Input: part model. Units: mm. Frame: model coordinates. A direction names the side the tool comes from. Coordinates: 2 decimals unless noted, no trailing zeros. Loops run counter-clockwise (first coordinate to the right, second up) from the corner with the lowest first, then second, coordinate; pieces in that order, holes last.
Autodesk Inventor part; units mm, degrees
ref_plane "YZ Plane" through (0, 0, 0) normal (1, 0, 0) x (0, 1, 0)
ref_plane "XZ Plane" through (0, 0, 0) normal (0, 1, 0) x (-1, 0, 0)
ref_plane "XY Plane" through (0, 0, 0) normal (0, 0, 1) x (1, 0, 0)
sketch "Sketch1" plane through (0, 0, 0) normal (0, 1, 0) x (-1, 0, 0)
  line L0 (400, -50) -> (400, 50)
  line L1 (400, 50) -> (390, 50)
  line L2 (390, 50) -> (390, -40)
  line L3 (390, -40) -> (300, -40)
  line L4 (300, -40) -> (300, -50)
  line L5 (300, -50) -> (400, -50)
  line L6 (250, -50) -> (250, -40)
  line L7 (250, -40) -> (150, -40)
  line L8 (150, -40) -> (150, -50)
  line L9 (150, -50) -> (250, -50)
  line L10 (100, -50) -> (100, -40)
  line L11 (100, -40) -> (10, -40)
  line L12 (10, -40) -> (10, 50)
  line L13 (10, 50) -> (0, 50)
  line L14 (0, 50) -> (0, -50)
  line L15 (0, -50) -> (100, -50)
  point P0 (0, 0)
  dimension "d0" = 100
  dimension "d1" = 100
  dimension "d2" = 10
  dimension "d3" = 10
  dimension "d4" = 100
  dimension "d5" = 100
  dimension "d6" = 100
  dimension "d7" = 10
  dimension "d8" = 10
  dimension "d9" = 50
  dimension "d10" = 50
  dimension "d11" = 400
  dimension "d12" = 50
  dimension "d13" = 50
extrude "Extrusion1" add sketch "Sketch1" along normal blind 100
sketch "Sketch2" plane through (0, 0, 0) normal (1, 0, 0) x (0, 1, 0)
  point P0 (0, 0)
sketch "Sketch3" plane through (0, 0, 50) normal (1, 0, 0) x (0, 0, -1)
  line L0 (92.5, 80) -> (97.5, 80)
  line L1 (97.5, 80) -> (97.5, 75)
  line L2 (97.5, 75) -> (92.5, 75)
  line L3 (92.5, 75) -> (92.5, 80)
  line L4 (97.5, 20) -> (92.5, 20)
  line L5 (92.5, 20) -> (92.5, 25)
  line L6 (92.5, 25) -> (97.5, 25)
  line L7 (97.5, 25) -> (97.5, 20)
  line L8 (0, 100) -> (100, 100)
  line L9 (100, 0) -> (100, 100)
  line L10 (0, 0) -> (100, 0)
  line L11 (92.5, 52.5) -> (97.5, 52.5)
  line L12 (97.5, 52.5) -> (97.5, 47.5)
  line L13 (97.5, 47.5) -> (92.5, 47.5)
  line L14 (92.5, 47.5) -> (92.5, 52.5)
  point P0 (50, 0)
  dimension "d16" = 20
  dimension "d17" = 5
  dimension "d18" = 5
  dimension "d19" = 2.5
  dimension "d20" = 20
  dimension "d21" = 5
  dimension "d22" = 5
  dimension "d24" = 7.5
  dimension "d25" = 5
  dimension "d26" = 5
  dimension "d27" = 2.5
  dimension "d28" = 22.5
extrude "Extrusion2" cut sketch "Sketch3" against normal blind 320
sketch "Sketch4" plane through (0, 0, 50) normal (1, 0, 0) x (0, 0, -1)
  line L0 (97.5, 75) -> (92.5, 75)
  line L1 (97.5, 80) -> (97.5, 75)
  line L2 (92.5, 80) -> (97.5, 80)
  line L3 (92.5, 75) -> (92.5, 80)
  line L4 (97.5, 47.5) -> (92.5, 47.5)
  line L5 (97.5, 52.5) -> (97.5, 47.5)
  line L6 (92.5, 52.5) -> (97.5, 52.5)
  line L7 (92.5, 47.5) -> (92.5, 52.5)
  line L8 (92.5, 25) -> (97.5, 25)
  line L9 (92.5, 20) -> (92.5, 25)
  line L10 (97.5, 20) -> (92.5, 20)
  line L11 (97.5, 25) -> (97.5, 20)
  line L12 (92.5, 80) -> (97.5, 80)
  line L13 (97.5, 80) -> (97.5, 75)
  line L14 (97.5, 75) -> (92.5, 75)
  line L15 (92.5, 75) -> (92.5, 80)
  line L16 (92.5, 52.5) -> (97.5, 52.5)
  line L17 (97.5, 52.5) -> (97.5, 47.5)
  line L18 (97.5, 47.5) -> (92.5, 47.5)
  line L19 (92.5, 47.5) -> (92.5, 52.5)
  line L20 (92.5, 25) -> (97.5, 25)
  line L21 (97.5, 25) -> (97.5, 20)
  line L22 (97.5, 20) -> (92.5, 20)
  line L23 (92.5, 20) -> (92.5, 25)
  point P0 (50, 0)
extrude "Extrusion3" add sketch "Sketch4" against normal blind 80
sketch "Sketch6" plane through (-250, 0, -40) normal (0, 0, 1) x (1, 0, 0)
  line L0 (-50, 80) -> (-50, 75)
  line L1 (-50, 80) -> (-70, 80)
  line L2 (-70, 80) -> (-70, 75)
  line L3 (-50, 75) -> (-70, 75)
  line L4 (-50, 52.5) -> (-50, 47.5)
  line L5 (-50, 52.5) -> (-70, 52.5)
  line L6 (-70, 52.5) -> (-70, 47.5)
  line L7 (-50, 47.5) -> (-70, 47.5)
  line L8 (-50, 25) -> (-50, 20)
  line L9 (-50, 25) -> (-70, 25)
  line L10 (-70, 25) -> (-70, 20)
  line L11 (-50, 20) -> (-70, 20)
  line L12 (0, 75) -> (0, 80)
  line L13 (100, 75) -> (0, 75)
  line L14 (100, 80) -> (100, 75)
  line L15 (100, 80) -> (0, 80)
  line L16 (0, 47.5) -> (0, 52.5)
  line L17 (100, 47.5) -> (0, 47.5)
  line L18 (100, 52.5) -> (100, 47.5)
  line L19 (100, 52.5) -> (0, 52.5)
  line L20 (0, 20) -> (0, 25)
  line L21 (100, 20) -> (0, 20)
  line L22 (100, 25) -> (100, 20)
  line L23 (100, 25) -> (0, 25)
  line L24 (170, 75) -> (170, 80)
  line L25 (170, 80) -> (150, 80)
  line L26 (150, 75) -> (150, 80)
  line L27 (170, 75) -> (150, 75)
  line L28 (170, 47.5) -> (170, 52.5)
  line L29 (170, 52.5) -> (150, 52.5)
  line L30 (150, 47.5) -> (150, 52.5)
  line L31 (170, 47.5) -> (150, 47.5)
  line L32 (170, 20) -> (170, 25)
  line L33 (170, 25) -> (150, 25)
  line L34 (150, 20) -> (150, 25)
  line L35 (170, 20) -> (150, 20)
  line L36 (-70, 80) -> (-60, 80)
  line L37 (-60, 80) -> (-60, 20)
  line L38 (-60, 20) -> (-70, 20)
  line L39 (-70, 20) -> (-70, 80)
  line L40 (10, 80) -> (90, 80)
  line L41 (90, 80) -> (90, 20)
  line L42 (90, 20) -> (10, 20)
  line L43 (10, 20) -> (10, 80)
  line L44 (160, 80) -> (170, 80)
  line L45 (170, 80) -> (170, 20)
  line L46 (170, 20) -> (160, 20)
  line L47 (160, 20) -> (160, 80)
  line L48 (0, 0) -> (0, 100)
  line L49 (100, 0) -> (100, 100)
  line L50 (10, 25) -> (90, 25)
  line L51 (90, 25) -> (90, 20)
  line L52 (90, 20) -> (10, 20)
  line L53 (10, 20) -> (10, 25)
  point P0 (250, 0)
  point P1 (160, 25)
  point P2 (160, 20)
  point P3 (160, 52.5)
  point P4 (160, 47.5)
  point P5 (160, 75)
  point P6 (10, 75)
  point P7 (90, 75)
  point P8 (90, 80)
  point P9 (10, 52.5)
  point P10 (10, 47.5)
  point P11 (90, 47.5)
  point P12 (90, 52.5)
  point P13 (10, 25)
  point P14 (10, 20)
  point P15 (-60, 25)
  point P16 (-60, 47.5)
  point P17 (-60, 52.5)
  point P18 (-60, 75)
  point P19 (90, 25)
  point P20 (90, 25)
  dimension "d33" = 10
  dimension "d34" = 10
extrude "Extrusion4" add sketch "Sketch6" against normal blind 10 contours L37 L3 L2 L1 | L37 L5 L39 L3 | L37 L7 L6 L5 | L37 L9 L39 L7 | L37 L11 L10 L9 | L43 L15 L41 L13 | L19 L41 L17 L43 | L23 L41 L21 L43 | L27 L47 L25 L24 | L45 L29 L47 L27 | L28 L31 L47 L29 | L45 L33 L47 L31 | L32 L35 L47 L33
sketch "Sketch8" plane through (0, 100, 0) normal (0, 1, 0) x (1, 0, 0)
  line L0 (-300, 50) -> (-400, 50)
  line L1 (-400, 50) -> (-400, -50)
  line L2 (-150, 40) -> (-150, 50)
  line L3 (-400, 50) -> (-150, 50)
  line L4 (-150, 50) -> (-150, -50)
  line L5 (-150, -50) -> (-400, -50)
  line L6 (-400, -50) -> (-400, 50)
  point P0 (0, 0)
  dimension "d44" = 250
  dimension "d45" = 100
extrude "Extrusion6" cut sketch "Sketch8" against normal through all
properties part number "Soccer Goal Split"
Item 1: Section query C-C (x = -83). Output: boundary loops of the cut face in (y, z).
Result:
outline: (0, -50) - (100, -50) - (100, -40) - (0, -40) - close
Item 2: Section query A-A (y = 69). Output: boundary loops of the cut face in (x, z).
Result:
outline: (-100, -50) - (0, -50) - (0, 50) - (-10, 50) - (-10, -40) - (-100, -40) - close
Item 3: Reachability of faces 1 (the face through (-95, 78, -47.5)), 2 (the face through (-10, 49, 4)), 3 (the face through (-28, 100, -41)) from +Z, -Z, +X, -X, +Y, -Y: full face, straight path, thin tool, end or side. Return the list, or none.
Result:
face 1: -X
face 2: +Z, -X, +Y, -Y
face 3: +Z, -Z, +X, -X, +Y
Item 4: Mould query, pull axis Z, two halves, no side actions, for faces 4 (the face through (-49, 49, -50)), 5 (the face through (-56, 49, -40)), 6 (the face through (0, 49, 1)), 7 (the face through (-95, 52.5, -45)). Classes: +Z half, -Z half, draft (parallel to the pull), parting line (faces both ways), or undercut.
Result:
face 4: -Z half
face 5: +Z half
face 6: draft
face 7: undercut
Item 5: Contact query for flat-ended pins moving along their axis: P1, Ø5.5, axis at x = -93, z = -46, coming from the -Y side; P2, Ø6, axis at y = 63, z = -22, coming from the -X side; P3, Ø4, axis at x = -95, y = 76.5, coming from the +Z side. Output: stop coordinate, or through.
Result:
P1: stops at y = 0
P2: stops at x = -10
P3: stops at z = -40
Item 6: Line query: L1, parallel to Z at x = -19.5, y = 91.5; L2, parallel to X at y = 32.5, z = -22. Output: solid intervals per line, ascending.
Result:
L1: z = -50 to -40
L2: x = -10 to 0
Item 7: Section query B-B (z = -36.5). Output: boundary loops of the cut face in (x, y).
Result:
outline: (-10, 0) - (0, 0) - (0, 100) - (-10, 100) - close
